The model under review builds one solid part; all positions refer to its coordinate system, in mm. A direction names the side the tool comes from. Give positions to 0.01 mm unless a question says otherwise; leave off trailing zeros. Loops run counter-clockwise (first coordinate to the right, second up) from the corner with the lowest first, then second, coordinate; pieces in that order, holes last. Notation, with made-up numbers: (84.25, 8.25) - (110.25, 8.25) arc R4 cw to (110.25, 14.25) - close; hole circle Ø11 at (10, -29). An arc over 180 degrees is marked (long way). Return JSON: item names as keys, results as strings. Group by question number.
```python
from build123d import *

# Parameters (mm, degrees)
EXTRUDE_1_DEPTH        = 45
SKETCH_2_R             = 1.5
CUT_EXTRUDE_1_DEPTH    = 5
PATTERN_LINEAR_1_COUNT = 2
PATTERN_LINEAR_1_PITCH = 40


with BuildPart() as part:
    # 草图1 → 凸台-拉伸1 (new body)
    with BuildSketch(Plane(origin=(0, 0, 0), x_dir=(1, 0, 0), z_dir=(0, 1, 0))):
        Polygon((4, 0), (2, 3.464101615), (-2, 3.464101615), (-4, 0), (-2, -3.464101615), (2, -3.464101615), align=None)
    extrude(amount=EXTRUDE_1_DEPTH)

    # 草图2 → 切除-拉伸1 (cut)
    with BuildSketch(Plane(origin=(0, 45, 0), x_dir=(1, 0, 0), z_dir=(0, 1, 0))):
        with Locations(Location((0, 0, 0), (0, 0, 270))):
            Circle(SKETCH_2_R)
    cut_extrude_1 = extrude(amount=-CUT_EXTRUDE_1_DEPTH, mode=Mode.SUBTRACT)

    # 阵列(线性)1: 切除-拉伸1 ×2
    with Locations(*[(0, -i * PATTERN_LINEAR_1_PITCH, 0) for i in range(1, PATTERN_LINEAR_1_COUNT)]):
        add(cut_extrude_1, mode=Mode.SUBTRACT)


solid = part.part
```
1) To check wall thickness, follow line 1 (X direction, y = 42.6, z = 0); line 2 (Y direction, x = -1.25, z = -0.5); line 3 (X direction, y = 38, z = -0.5). State the ranges of each line that lie inside material, in increasing order.
2) We need section B-B, the plane y = 28.5. Write out the cut boundary in (x, z), plus the area to 3 significant figures.
3) Tool access review of faces 4 (the face through (0, 5, 0)), 5 (the face through (0, 22, 3.464)), 6 (the face through (0, 40, 0)): name each direction out of +Z, -Z, +X, -X, +Y, -Y from which nothing blocks a thin tool from reaching the whole face with its end or side.
4) We need section A-A, the plane x = 0. Write out the cut boundary in (y, z).
5) We need section D-D, the plane z = 3. Write out the cut boundary in (x, y).
6) We need section C-C, the plane z = -0.75. Write out the cut boundary in (x, y).
7) Draft analysis for pull direction Z (two halves, no side actions). For faces 1 (the face through (0.45, 42.54, 1.43)), 2 (the face through (0, 0, -2)), 3 (the face through (0, 22, -3.464)), state which applies: +Z half, -Z half, draft (parallel to the pull), parting line (faces both ways), or undercut.
8) For pin 1 Ø1 at (y, z) = (34.5, -2.5) entering from -X; pin 2 Ø1.5 at (x, z) = (-0.5, 0.5) entering from +Y; pin 3 Ø0.9 at (x, z) = (0.5, 0.5) entering from -Y, all flat-tipped, find the tip position at first contact; note any pin that passes through.
Findings:
{
 "1": {"line 1": "x = -4 to -1.5, 1.5 to 4", "line 2": "y = 5 to 40", "line 3": "x = -3.71 to 3.71"},
 "2": {"outline": "(-4, 0) - (-2, -3.46) - (2, -3.46) - (4, 0) - (2, 3.46) - (-2, 3.46) - close", "area": "41.6 mm^2"},
 "3": {"face 4": "-Y", "face 5": "+Z, +X, -X, +Y, -Y", "face 6": "+Y"},
 "4": {"outline": "(0, -3.46) - (45, -3.46) - (45, -1.5) - (40, -1.5) - (40, 1.5) - (45, 1.5) - (45, 3.46) - (0, 3.46) - (0, 1.5) - (5, 1.5) - (5, -1.5) - (0, -1.5) - close"},
 "5": {"outline": "(-2.27, 0) - (2.27, 0) - (2.27, 45) - (-2.27, 45) - close"},
 "6": {"outline": "(-3.57, 0) - (-1.3, 0) - (-1.3, 5) - (1.3, 5) - (1.3, 0) - (3.57, 0) - (3.57, 45) - (1.3, 45) - (1.3, 40) - (-1.3, 40) - (-1.3, 45) - (-3.57, 45) - close"},
 "7": {"face 1": "undercut", "face 2": "draft", "face 3": "-Z half"},
 "8": {"pin 1": "stops at x = -2.85", "pin 2": "stops at y = 40", "pin 3": "stops at y = 5"}
}
